Design review of the part built by this model. Coordinates are the model's own, in mm. A direction names the side the tool comes from. Coordinates: 2 decimals unless noted, no trailing zeros. Order: outer loops, then holes, each group sorted by start corner. A loop starts at its lowest first (then second) coordinate and runs counter-clockwise, first axis right, second up. Notation, with made-up numbers: (30.25, 7) -> (52.25, 7) arc R12 cw to (52.25, 26) -> close; hole circle Ø7 at (-19, 1.25). An arc over 180 degrees is marked (long way). Write item = value, one per line.
```python
from build123d import *

# Parameters (mm, degrees)
SKETCH3_W             = 50.5
SKETCH3_H             = 101
SKETCH3_W_2           = 48.5
SKETCH3_H_2           = 99
BOSS_EXTRUDE1_DEPTH   = 1600
BOSS_EXTRUDE1_2_DEPTH = 1600
SKETCH8_R             = 39.5
CUT_EXTRUDE1_DEPTH    = 2500
SKETCH9_R             = 40.5
CUT_EXTRUDE2_DEPTH    = 1
SKETCH10_R            = 40.5
CUT_EXTRUDE3_DEPTH    = 1
SKETCH13_R            = 40.5
SKETCH13_R_2          = 39.5
BOSS_EXTRUDE2_DEPTH   = 2497


with BuildPart() as part:
    # Sketch3 → Boss-Extrude1 (new body)
    with BuildSketch(Plane(origin=(0, 0, 0), x_dir=(1, 0, 0), z_dir=(0, 1, 0))):
        with Locations((-25.25, 0)):
            Rectangle(SKETCH3_W, SKETCH3_H)
        with Locations((-25.25, 0)):
            Rectangle(SKETCH3_W_2, SKETCH3_H_2, mode=Mode.SUBTRACT)
    extrude(amount=BOSS_EXTRUDE1_DEPTH)


with BuildPart() as body_2:
    # Sketch3 → Boss-Extrude1 2 (new body)
    with BuildSketch(Plane(origin=(0, 0, 0), x_dir=(1, 0, 0), z_dir=(0, 1, 0))):
        with Locations((2423.25, 0)):
            Rectangle(SKETCH3_W, SKETCH3_H)
        with Locations((2423.25, 0)):
            Rectangle(SKETCH3_W_2, SKETCH3_H_2, mode=Mode.SUBTRACT)
    extrude(amount=BOSS_EXTRUDE1_2_DEPTH)


with BuildPart() as cut_extrude1_tool:
    # Sketch8 → Cut-Extrude1 (new body, through all)
    with BuildSketch(Plane.ZY.offset(50.5)):
        with Locations((0, 50)):
            Circle(SKETCH8_R)
        with Locations((0, 1550)):
            Circle(SKETCH8_R)
    extrude(amount=-CUT_EXTRUDE1_DEPTH)


with BuildPart() as part_1:
    add(part.part)

    # Cut-Extrude1: cut by cut_extrude1_tool
    add(cut_extrude1_tool.part, mode=Mode.SUBTRACT)

    # Sketch9 → Cut-Extrude2 (cut)
    with BuildSketch(Plane(origin=(0, 0, 0), x_dir=(0, 0, -1), z_dir=(1, 0, 0))):
        with Locations((0, 50)):
            Circle(SKETCH9_R)
        with Locations((0, 1550)):
            Circle(SKETCH9_R)
    extrude(amount=-CUT_EXTRUDE2_DEPTH, mode=Mode.SUBTRACT)



with BuildPart() as body_2_1:
    add(body_2.part)

    # Cut-Extrude1: cut by cut_extrude1_tool
    add(cut_extrude1_tool.part, mode=Mode.SUBTRACT)

    # Sketch10 → Cut-Extrude3 (cut)
    with BuildSketch(Plane.ZY.offset(-2398)):
        with Locations((0, 50)):
            Circle(SKETCH10_R)
        with Locations((0, 1550)):
            Circle(SKETCH10_R)
    extrude(amount=-CUT_EXTRUDE3_DEPTH, mode=Mode.SUBTRACT)


with BuildPart() as part_2:
    add(part_1.part)

    add(body_2_1.part)  # Boss-Extrude2 merges body 2
    # Sketch13 → Boss-Extrude2 (add)
    with BuildSketch(Plane.ZY.offset(-2447.5)):
        with Locations((0, 50)):
            Circle(SKETCH13_R)
        with Locations((0, 50)):
            Circle(SKETCH13_R_2, mode=Mode.SUBTRACT)
        with Locations((0, 1550)):
            Circle(SKETCH13_R)
        with Locations((0, 1550)):
            Circle(SKETCH13_R_2, mode=Mode.SUBTRACT)
    extrude(amount=BOSS_EXTRUDE2_DEPTH)


solid = part_2.part
```
(1) Insertion check: pin 1 (3 mm diameter, centred on x = 2165, z = -2, fed in from -Y); pin 2 (1 mm diameter, centred on x = 411.5, z = 29, fed in from -Y) (3 decimals); pin 3 (1 mm diameter, centred on x = 828, z = -6, fed in from +Y). Each pin has a flat end and moves straight along its axis. Give the tip position at first contact, or say it passes through.
Report:
pin_1 = 9.5
pin_2 = 21.225
pin_3 = 1590.12
(2) We need section D-D (x = 476). Write out the cut boundary in (y, z).
Report:
outline = circle Ø81 at (50, 0); circle Ø81 at (1550, 0); hole circle Ø79 at (50, 0); hole circle Ø79 at (1550, 0)
(3) The part is to be moulded in two halves that separate along X. For faces 1 (the flat face through (2423, 789, 49.5)), 2 (the flat face through (2423, 789, -50.5)), 3 (the flat face through (-50.5, 789, 1)), say which applies: released by +X, released by -X, zero draft, split by the parting line, or undercut.
Report:
face_1 = undercut
face_2 = zero draft
face_3 = released by -X
(4) We need section A-A (y = 50). Give the number of separate pieces and of enclosed holes in the cut face, and give its area (3 significant figures).
Report:
separate_pieces = 2
enclosed_holes = 4
area = 5,270 mm²
(5) For L1, parallel to Y at x = 1871, z = 0; L2, parallel to X at y = 510, z = 24.5; L3, parallel to Y at x = 2448.15, z = 0, list the stretches that pass through material, from the lowest coordinate up.
Report:
L1 = 9.5 to 10.5, 89.5 to 90.5, 1509.5 to 1510.5, 1589.5 to 1590.5
L2 = -50.5 to -49.5, -1 to 0, 2398 to 2399, 2447.5 to 2448.5
L3 = 0 to 10.5, 89.5 to 1510.5, 1589.5 to 1600
(6) For faces 4 (the flat face through (2423, 789, -49.5)), 5 (the flat face through (-50, 1600, 0)), 6 (the flat face through (2399, 789, 1)), list the 3-axis set-ups (+Z, -Z, +X, -X, +Y, -Y) from which the entire face can be reached by the end or side of a thin tool; tool diameter is ignored.
Report:
face_4 = +Y, -Y
face_5 = +Z, -Z, +X, -X, +Y
face_6 = none
(7) We need section B-B (y = 676.5). Write out the cut boundary in (x, z).
Report:
outline = (-50.5, -50.5) -> (0, -50.5) -> (0, 50.5) -> (-50.5, 50.5) -> close; (2398, -50.5) -> (2448.5, -50.5) -> (2448.5, 50.5) -> (2398, 50.5) -> close; hole (-49.5, -49.5) -> (-1, -49.5) -> (-1, 49.5) -> (-49.5, 49.5) -> close; hole (2399, -49.5) -> (2447.5, -49.5) -> (2447.5, 49.5) -> (2399, 49.5) -> close
